Can you work these out from the model? Positions are in its coordinate system, mm. A direction names the side the tool comes from. Coordinates: 2 decimals unless noted, no trailing zeros. Loops run counter-clockwise (first coordinate to the right, second up) from the corner with the lowest first, then second, coordinate; pieces in that order, holes last. Notation, with made-up numbers: (2.5, 16.5) - (7.5, 16.5) arc R18 ccw to (7.5, 24.5) - close; hole circle Ø10 at (26.25, 42). An arc over 180 degrees is marked (long way). Put each result on its own line as item: value. Start each with the question number.
Autodesk Fusion 360 part; units mm, degrees
sketch "Sketch1" plane through (0, 0, 0) normal (0, 1, 0) x (1, 0, 0)
  line L0 (10, -10) -> (118, -10)
  line L1 (148, -40) -> (148, -40)
  line L2 (118, -70) -> (10, -70)
  line L3 (10, -70) -> (10, -10)
  arc A0 (148, -40) -> (118, -10) centre (118, -40) ccw
  arc A1 (118, -70) -> (148, -40) centre (118, -40) ccw
  circle A2 centre (118, -40) radius 13
  point P0 (148, -10)
  dimension "d1" = 138
  dimension "d2" = 60
  dimension "d3" = 30
  dimension "d4" = 30
  dimension "d5" = 26
extrude "Extrude1" add sketch "Sketch1" along normal blind 20
sketch "Sketch2" plane through (0, 20, 0) normal (0, 1, 0) x (-1, 0, 0)
  circle A0 centre (-118, 40) radius 13
  line L0 (-10, 70) -> (-118, 70)
  arc A1 (-118, 70) -> (-118, 10) centre (-118, 40) ccw
  line L1 (-118, 10) -> (-10, 10)
  line L2 (-10, 10) -> (-10, 70)
  line L3 (-118, 47) -> (-155, 47)
  arc A2 (-155, 47) -> (-155, 33) centre (-155, 40) ccw
  line L4 (-155, 33) -> (-118, 33)
  arc A3 (-118, 33) -> (-118, 47) centre (-118, 40) ccw
  line L5 (-118, 40) -> (-155, 40) construction
  dimension "d8" = 14
extrude "Extrude2" cut sketch "Sketch2" against normal blind 10 contours A0 A1 L3 L4
sketch "Sketch4" plane through (0, 20, 0) normal (0, 1, 0) x (-1, 0, 0)
  line L0 (-147.1719, 47) -> (-128.9545, 47)
  arc A0 (-128.9545, 33) -> (-128.9545, 47) centre (-118, 40) ccw
  line L1 (-128.9545, 33) -> (-147.1719, 33)
  arc A1 (-147.1719, 33) -> (-118, 10) centre (-118, 40) ccw
  line L2 (-118, 10) -> (-10, 10)
  line L3 (-10, 10) -> (-10, 70)
  line L4 (-10, 70) -> (-118, 70)
  arc A2 (-118, 70) -> (-147.1719, 47) centre (-118, 40) ccw
  line L5 (-10, 70) -> (-70, 70) construction
  line L6 (-70, 70) -> (-70, 10) construction
  line L7 (-70, 70) -> (-40.3015, 40.3015) construction
  line L8 (-70, 70) -> (-28, 70) construction
  line L9 (-70, 70) -> (-40.3015, 40.3015)
  line L10 (-40.3015, 40.3015) -> (-70, 10.603)
  line L11 (-70, 10.603) -> (-99.6985, 40.3015)
  line L12 (-99.6985, 40.3015) -> (-70, 70)
  dimension "d11" = 60
  dimension "d12" = 45
  dimension "d13" = 42
  dimension "d14" = 42
extrude "Extrude3" add sketch "Sketch4" along normal blind 56 contours L9 L10 L11 L12
hole "Hole1" at (70, 76, 40.3015) direction (0, -1, 0) diameter 30 depth 90 tip angle 180
hole "Hole2" at (70, 0, 40.3015) direction (0, 1, 0) diameter 50 depth 10 tip angle 180
sketch "Sketch5" plane through (0, 20, 0) normal (0, 1, 0) x (-1, 0, 0)
  line L0 (-147.1719, 47) -> (-128.9545, 47)
  arc A0 (-128.9545, 33) -> (-128.9545, 47) centre (-118, 40) ccw
  line L1 (-128.9545, 33) -> (-147.1719, 33)
  arc A1 (-147.1719, 33) -> (-118, 10) centre (-118, 40) ccw
  line L2 (-118, 10) -> (-10, 10)
  line L3 (-10, 10) -> (-10, 70)
  line L4 (-10, 70) -> (-70, 70)
  line L5 (-70, 70) -> (-40.3015, 40.3015)
  line L6 (-40.3015, 40.3015) -> (-70, 10.603)
  line L7 (-70, 10.603) -> (-99.6985, 40.3015)
  line L8 (-99.6985, 40.3015) -> (-70, 70)
  line L9 (-70, 70) -> (-118, 70)
  arc A2 (-118, 70) -> (-147.1719, 47) centre (-118, 40) ccw
  line L10 (-10, 57) -> (-10, 63)
  line L11 (-10, 63) -> (-20, 63)
  line L12 (-20, 51) -> (-10, 51)
  arc A3 (-10, 51) -> (-10, 63) centre (-10, 57) ccw
  line L13 (-10, 63) -> (-20, 63)
  arc A4 (-20, 63) -> (-20, 51) centre (-20, 57) ccw
  line L14 (-20, 57) -> (-10, 57) construction
  dimension "d24" = 6
  dimension "d25" = 10
extrude "Extrude4" cut sketch "Sketch5" against normal blind 20 contours L3 L10 L11 L12 L13 A4
sketch "Sketch6" plane through (0, 20, 0) normal (0, 1, 0) x (-1, 0, 0)
  line L0 (-20, 63) -> (-10, 63)
  line L1 (-10, 63) -> (-10, 70)
  line L2 (-10, 70) -> (-70, 70)
  line L3 (-70, 70) -> (-40.3015, 40.3015)
  line L4 (-40.3015, 40.3015) -> (-70, 10.603)
  line L5 (-70, 10.603) -> (-99.6985, 40.3015)
  line L6 (-99.6985, 40.3015) -> (-70, 70)
  line L7 (-70, 70) -> (-118, 70)
  arc A0 (-118, 70) -> (-147.1719, 47) centre (-118, 40) ccw
  line L8 (-147.1719, 47) -> (-128.9545, 47)
  arc A1 (-128.9545, 33) -> (-128.9545, 47) centre (-118, 40) ccw
  line L9 (-128.9545, 33) -> (-147.1719, 33)
  arc A2 (-147.1719, 33) -> (-118, 10) centre (-118, 40) ccw
  line L10 (-118, 10) -> (-10, 10)
  line L11 (-10, 10) -> (-10, 51)
  line L12 (-10, 51) -> (-20, 51)
  arc A3 (-20, 63) -> (-20, 51) centre (-20, 57) ccw
  line L13 (-10, 10) -> (-40, 10)
  line L14 (-40, 10) -> (-40, 25)
  line L15 (-40, 25) -> (-10, 25)
  line L16 (-10, 25) -> (-10, 10)
  dimension "d28" = 30
  dimension "d29" = 15
extrude "Extrude5" add sketch "Sketch6" along normal blind 37 contours L10 L11 L13 L14 L15 L16
fillet "Fillet1" radius 15 2 edges at (10, 57, 17.5) (40, 57, 17.5)
hole "Hole3" at (25, 42, 25) direction (0, 0, -1) diameter 20 depth 130 tip angle 180
Q1. I want a section at B-B on z = 31.5. List the corners of the cut face in (x, y) for me.
Q2. We'd pull the mould along Z, two halves only. Please class faces 5 (the flat face through (138, 15, 33)), 6 (the flat face through (25, 30, 25)), 7 (the cylindrical face through (25, 52, 17)), 8 (the cylindrical face through (26, 10, 57)): released by +Z, released by -Z, zero draft, split by the parting line, or undercut.
Q3. I want a section at A-A on y = 15. List the corners of the cut face in (x, z) for me, and give its area (3 significant figures).
Q4. I want a section at C-C on x = 111. List the corners of the cut face in (y, z) for me, and give its area (3 significant figures).
Q5. Will these pins go through, and if not, where does the flat tip stop? pin 1 (18 mm diameter, centred on x = 107.5, z = 27, fed in from +Y); pin 2 (18 mm diameter, centred on x = 25, y = 42, fed in from +Z); pin 3 (12 mm diameter, centred on y = 55, z = 22, fed in from +X); pin 4 (11 mm diameter, centred on x = 141.5, y = 14, fed in from +Z).
Q6. I want a section at D-D on z = 57. List the corners of the cut face in (x, y) for me.
Q7. Please list where these lines run through material, in increasing order: line 1 along Z through (x, y) = (118, 8.75); line 2 along Z through (x, y) = (70, 42); line 3 along X through (y, z) = (8, 40). Write a range as [from, to].
Q8. On a 3-axis mill with a long thin cutter (end or side, diameter ignored), from which of +Z, -Z, +X, -X, +Y, -Y can I reach the whole of each face in a straight line? I mean faces 1 (the cylindrical face through (45.213, 5.07, 43.556)), 2 (the flat face through (54.943, 47.608, 25.66)), 3 (the flat face through (138, 15, 47)), 4 (the flat face through (84.641, 47.608, 25.244)). Say none if no direction works.
Calculated:
1. outline: (10, 0) - (46.6, 0) - (46.6, 10) - (57.85, 10) - (57.85, 76) - (49.1, 76) - (49.1, 20) - (10, 20) - close; (82.15, 10) - (93.4, 10) - (93.4, 0) - (108.16, 0) - (108.16, 20) - (90.9, 20) - (90.9, 76) - (82.15, 76) - close; (127.84, 0) - (146.77, 0) - (146.77, 20) - (127.84, 20) - close
2. face 5: undercut
2. face 6: released by +Z
2. face 7: zero draft
2. face 8: undercut
3. outline: (10, 10) - (118, 10) arc R30 ccw to (147.17, 33) - (128.95, 33) arc R13 cw (long way) to (128.95, 47) - (147.17, 47) arc R30 ccw to (118, 70) - (10, 70) - (10, 63) - (20, 63) arc R6 cw to (20, 51) - (10, 51) - close; hole circle Ø30 at (70, 40.3)
3. area: 6,240 mm2
4. outline: (0, 10) - (20, 10) - (20, 29.05) - (0, 29.05) - close; (0, 50.95) - (20, 50.95) - (20, 70) - (0, 70) - close
4. area: 762 mm2
5. pin 1: y = 20
5. pin 2: through
5. pin 3: x = 87.4
5. pin 4: z = 64
6. outline: (26, 0) - (51.39, 0) - (51.39, 10) - (88.61, 10) - (88.61, 0) - (142.72, 0) - (142.72, 20) - (83, 20) - (83, 76) - (57, 76) - (57, 20) - (26, 20) - close
7. line 1: [10, 27], [53, 70]
7. line 2: [10.6, 25.3], [55.3, 70]
7. line 3: [10, 45], [95, 105], [131, 148]
8. face 1: -Y
8. face 2: -Z, +Y
8. face 3: +X, +Y
8. face 4: -Z, +X, +Y
